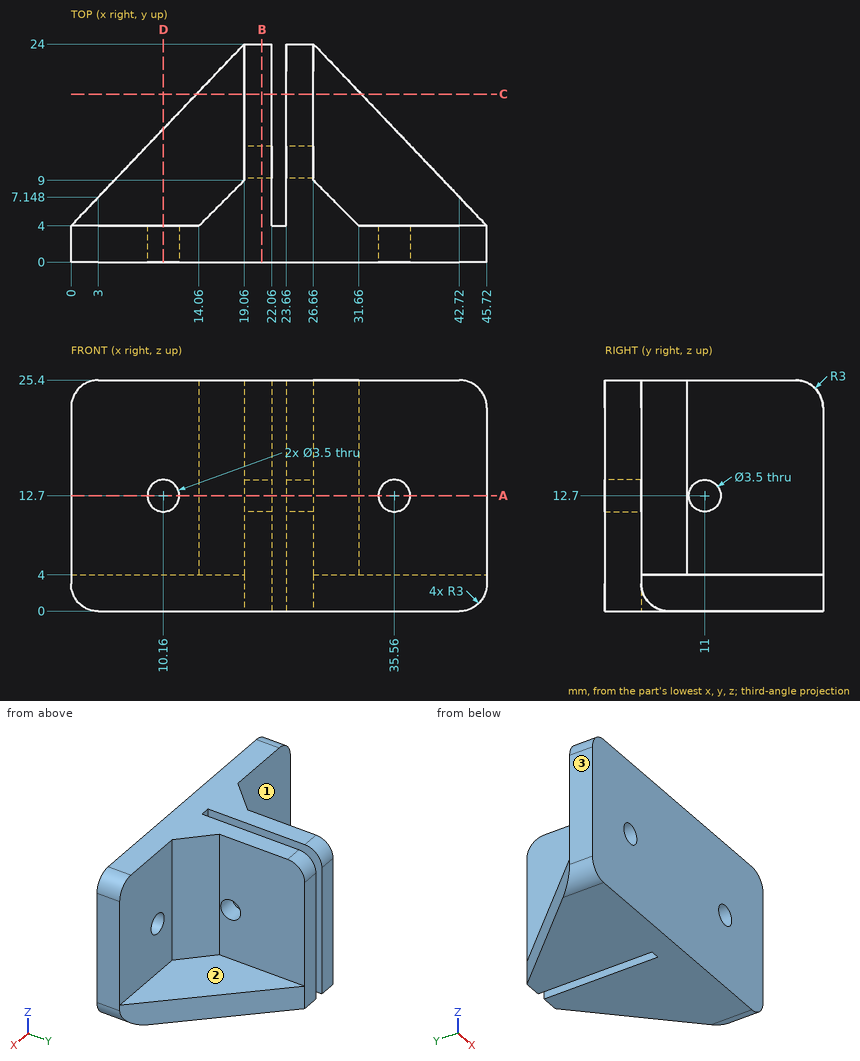
Geometry check sheet. Reference: drawing and pictorial views, mm from the part's lowest x, y, z. A direction names the side the tool comes from. Round coordinates to 2 decimals unless told otherwise and drop trailing zeros. Order: outer loops, then holes, each group sorted by start corner. A loop starts at its lowest first (then second) coordinate and runs counter-clockwise, first axis right, second up. Notation, with made-up numbers: (1, 40.25) - (59, 40.25) arc R12 cw to (59, 61.25) - close; hole circle Ø10 at (68.25, 74). An arc over 180 degrees is marked (long way). Write item = value, one per line.
Q1. Thickness scan on line 1 along X through (y, z) = (1.25, 12.7); line 2 along X through (y, z) = (15.25, 17.75); line 3 along Y through (x, z) = (21.05, 12.7). Record the ranges inside material, lowest first.
Computed:
line_1 = 0 to 8.41, 11.91 to 33.81, 37.31 to 45.72
line_2 = 19.06 to 22.06, 23.66 to 26.66
line_3 = 0 to 9.25, 12.75 to 24
Q2. Section check A-A (z = 12.7). State how many separate pieces and enclosed holes the cut face has, and give its area (3 significant figures).
Computed:
separate_pieces = 5
enclosed_holes = 0
area = 279 mm^2
Q3. Go/stop test with flat-tipped pins: pin 1 (5.5 mm diameter, centred on x = 7.5, y = 15, fed in from +Z); pin 2 (5.5 mm diameter, centred on y = 11, z = 12.7, fed in from +X); pin 3 (2 mm diameter, centred on x = 36.5, z = 2.5, fed in from +Y). Record where each tip stops, or that it passes through.
Computed:
pin_1 = 4
pin_2 = 27.41
pin_3 = 14.72
Q4. Section check B-B (x = 21). Record the boundary of the cut face in (y, z), and give its area (3 significant figures).
Computed:
outline = (0, 0) - (24, 0) - (24, 22.4) arc R3 ccw to (21, 25.4) - (0, 25.4) - close; hole circle Ø3.5 at (11, 12.7)
area = 598 mm^2
Q5. Tool access check on the marked faces 1, 2 and 3. Record the directions out of +Z, -Z, +X, -X, +Y, -Y that give a thin tool (end or side, any length) a straight path to the whole face; none if there is none.
Computed:
face_1 = +Z, -X, +Y
face_2 = +Z, +X, +Y
face_3 = +Z, -Z, -X, +Y, -Y
Q6. Section check D-D (x = 10.16). Record the boundary of the cut face in (y, z).
Computed:
outline = (0, 0) - (14.66, 0) - (14.66, 4) - (4, 4) - (4, 10.95) - (0, 10.95) - close; (0, 14.45) - (4, 14.45) - (4, 25.4) - (0, 25.4) - close
Q7. Section check C-C (y = 18.5). Record the boundary of the cut face in (x, z), and give its area (3 significant figures).
Computed:
outline = (13.82, 0) - (22.06, 0) - (22.06, 25.4) - (19.06, 25.4) - (19.06, 4) - (13.82, 4) - close; (23.66, 0) - (31.9, 0) - (31.9, 4) - (26.66, 4) - (26.66, 25.4) - (23.66, 25.4) - close
area = 194 mm^2
